Source: CAD feature listing. Evaluate the final solid. Frame: model axes, mm. Face numbers are marked on the shaded views. A direction names the side the tool comes from. Coordinates: 2 decimals unless noted, no trailing zeros. Write each loop counter-clockwise with the first axis right and the second up, starting at its lowest first coordinate (ties: lowest second). Pieces come first, ordered by that corner, then holes. Notation, with made-up numbers: M 36,7.25 L 65,7.25 A17 ccw 65,26.25 Z; hole C 11.5,49.5 d8. An arc over 180 degrees is marked long. One line per item, written item: value. Start each with the question number.
Item 1: Cut plane A-A, the plane z = 3. Output: boundary loops of the cut face in (x, y), then the cut area to 3 significant figures.
Item 2: Cut plane B-B, the plane y = 8. Output: boundary loops of the cut face in (x, z).
Item 3: Pin query (flat end, axial travel): P1, Ø4, axis at x = -1, z = -5, coming from the -Y side; P2, Ø10, axis at y = -6.5, z = -1, coming from the +X side; P3, Ø2.5, axis at x = 2, z = 3, coming from the +Y side; P4, Ø3, axis at x = -3, y = -29, coming from the -Z side. Return the tip coordinate at first contact, or that it passes through.
Item 4: Ray query, L1, parallel to X at y = 33.95, z = 0; L2, parallel to Y at x = -1, z = 1.75; L3, parallel to Z at x = 0.5, y = -2.5. Return the intervals inside material, ascending. Write a range as from..to.
Item 5: Set-up query: the marked faces 3 and 4. Return all of +Z, -Z, +X, -X, +Y, -Y with unobstructed straight access to the full face (end or side cutting, diameter ignored); none if empty.
Item 6: Mould query, pull axis X, two halves, no side actions, for the marked faces 1 and 2. Classes: released by +X, released by -X, zero draft, split by the parting line, or undercut.
```python
from build123d import *

# Parameters (mm, degrees)
F0_R      = 10
F0_R_2    = 9.15
F1_DEPTH  = 32.5
F3_R      = 10
F4_DEPTH  = 2
F6_R      = 10
F7_DEPTH  = 2
F9_W      = 20.5420348992
F9_H      = 75
F9_W_2    = 19.674062295
F10_DEPTH = 25
F12_DEPTH = 25
F13_R     = 0.5
F14_DEPTH = 80
F15_R     = 2
F15_R_2   = 1
F16_DEPTH = 4
F17_R     = 2
F17_R_2   = 1
F18_DEPTH = 4


with BuildPart() as f1:
    # F0 (on Front) → F1 (new body, symmetric)
    with BuildSketch(Plane.XZ):
        Circle(F0_R)
        Circle(F0_R_2, mode=Mode.SUBTRACT)
    extrude(amount=F1_DEPTH, both=True)

    # F3 (on face) → F4 (join)
    with BuildSketch(Plane.XZ.offset(32.5)):
        Circle(F3_R)
    extrude(amount=F4_DEPTH)

    # F6 (on face) → F7 (join)
    with BuildSketch(Plane(origin=(0, 32.5, 0), x_dir=(-1, 0, 0), z_dir=(0, 1, 0))):
        Circle(F6_R)
    extrude(amount=F7_DEPTH)

    # F9 (on offset) → F10 (cut)
    with BuildSketch(Plane.XY.offset(11)):
        with Locations((-14.2710174496, 0)):
            Rectangle(F9_W, F9_H)
        with Locations((13.8370311475, 0)):
            Rectangle(F9_W_2, F9_H)
    extrude(amount=-F10_DEPTH, mode=Mode.SUBTRACT)

    # F11 (on face) → F12 (cut)
    with BuildSketch(Plane.YZ.offset(4)):
        with BuildLine():
            Line((-32.5, -0.2), (-32.5, 0.2))
            ThreePointArc((-32.5, 0.2), (-32.9, 0), (-32.5, -0.2))
        make_face()
        with BuildLine():
            ThreePointArc((32.9, 0), (32.7618033989, 0.2236067977), (32.5, 0.2))
            Line((32.5, 0.2), (32.5, -0.2))
            ThreePointArc((32.5, -0.2), (32.7618033989, -0.2236067977), (32.9, 0))
        make_face()
    extrude(amount=-F12_DEPTH, mode=Mode.SUBTRACT)

    # F13 (on face) → F14 (cut)
    with BuildSketch(Plane(origin=(0, 34.5, 0), x_dir=(-1, 0, 0), z_dir=(0, 1, 0))):
        with Locations((-2, 0)):
            Circle(F13_R)
        with Locations((2, 0)):
            Circle(F13_R)
    extrude(amount=-F14_DEPTH, mode=Mode.SUBTRACT)

    # F15 (on Right) → F16 (join)
    with BuildSketch(Plane.YZ):
        with Locations((36, -8)):
            Circle(F15_R)
        with Locations((36, -8)):
            Circle(F15_R_2, mode=Mode.SUBTRACT)
    extrude(amount=F16_DEPTH)

    # F17 (on Right) → F18 (join)
    with BuildSketch(Plane.YZ):
        with Locations((-36, 8)):
            Circle(F17_R)
        with Locations((-36, 8)):
            Circle(F17_R_2, mode=Mode.SUBTRACT)
    extrude(amount=F18_DEPTH)


solid = f1.part
```
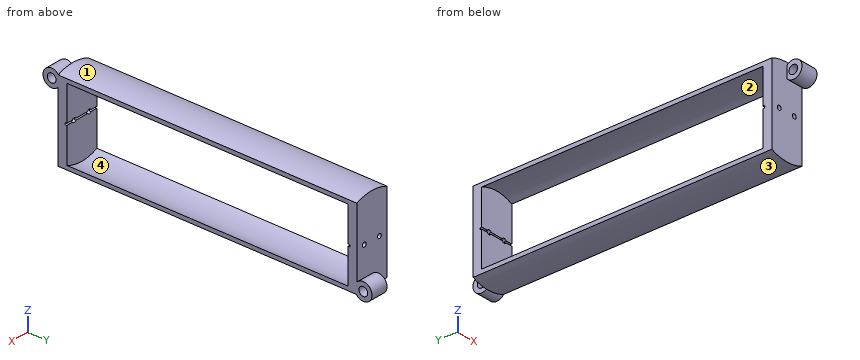
From the geometry:
1. outline: M -4,-34.5 L 4,-34.5 L 4,-32.5 L -4,-32.5 Z; M -4,32.5 L 4,32.5 L 4,34.5 L -4,34.5 Z
1. area: 32.0 mm²
2. outline: M -4,-9.17 A10 ccw 4,-9.17 L 4,-8.23 A9.15 cw -4,-8.23 Z; M -4,8.23 A9.15 cw 4,8.23 L 4,9.17 A10 ccw -4,9.17 Z
3. P1: stops at y = -34.5
3. P2: passes through
3. P3: stops at y = 34.5
3. P4: stops at z = -9.89
4. L1: x = -4..-2.5, -1.5..1.5, 2.5..4
4. L2: y = -34.5..-32.5, 32.5..34.5
4. L3: z = -9.99..-9.14, 9.14..9.99
5. face 3: -Z, -Y
5. face 4: none
6. face 1: split by the parting line
6. face 2: undercut
